from build123d import *

# Parameters (mm, degrees)
SKETCH_1_R           = 47
EXTRUDE_1_DEPTH      = 25
SKETCH_2_R           = 78
EXTRUDE_2_DEPTH      = 24
SKETCH_3_R           = 56
EXTRUDE_3_DEPTH      = 30
EXTRUDE_4_DEPTH      = 60
EXTRUDE_4_DEPTH_BACK = 60
SKETCH_4_R           = 58
SKETCH_4_R_2         = 38


with BuildPart() as part:
    # 草图1 → 凸台-拉伸1 (new body)
    with BuildSketch(Plane.XY):
        Circle(SKETCH_1_R)
    extrude(amount=-EXTRUDE_1_DEPTH)

    # 草图2 → 凸台-拉伸2 (add)
    with BuildSketch(Plane.XY):
        Circle(SKETCH_2_R)
    extrude(amount=EXTRUDE_2_DEPTH)

    # 草图3 → 凸台-拉伸3 (add)
    with BuildSketch(Plane.XY):
        Circle(SKETCH_3_R)
    extrude(amount=EXTRUDE_3_DEPTH)

    # 草图4 → 凸台-拉伸4 (add, two sides: drawn at the far end of the back side and taken through both)
    with BuildSketch(Plane(origin=(0, 0, 0), x_dir=(1, 0, 0), z_dir=(0, 1, 0)).offset(-EXTRUDE_4_DEPTH_BACK)):
        with Locations((0, -60)):
            Circle(SKETCH_4_R)
        with Locations((0, -60)):
            Circle(SKETCH_4_R_2, mode=Mode.SUBTRACT)
    extrude(amount=EXTRUDE_4_DEPTH + EXTRUDE_4_DEPTH_BACK)


solid = part.part
Build history of the part. All positions in model axes, mm. A direction names the side the tool comes from. Give positions to 0.01 mm unless a question says otherwise; leave off trailing zeros. Write each loop counter-clockwise with the first axis right and the second up, starting at its lowest first coordinate (ties: lowest second). Pieces come first, ordered by that corner, then holes. Notation, with made-up numbers: (-23, -4) - (7, -4) arc R15 ccw to (7, 22) - close; hole circle Ø11 at (84, -24.5). An arc over 180 degrees is marked (long way). Use one line per item in the form item = value. Start each with the question number.
1. Probe line 1 (X direction, y = 30.5, z = 60); line 2 (Z direction, x = 0, y = -32.5); line 3 (X direction, y = -57.5, z = 29). List the from-to ranges inside material, lowest first. Write a range as [from, to].
2. Band-saw the part on C-C on x = 0. Write the cut outline in (y, z).
3. Band-saw the part on D-D on x = -19. Write the cut outline in (y, z).
4. Drop flat-ended pins along their axis: pin 1 Ø3 at (x, y) = (-51, -4.5) entering from +Z; pin 2 Ø5 at (y, z) = (44.5, 83.5) entering from +X; pin 3 Ø3 at (y, z) = (-20, 12.5) entering from +X. Give the stop position or say it passes through.
5. 3-axis set-ups, long thin cutter, end or side, ignore diameter. For faces 1 (the face through (56, 0, 27)), 2 (the face through (-56, 0, 27)), 3 (the face through (0, 1, 30)): which of +Z, -Z, +X, -X, +Y, -Y reach the whole face in a straight line?
6. Band-saw the part on B-B on y = 0. Write the cut outline in (x, z).
7. Band-saw the part on A-A on z = 60. Write the cut outline in (x, y).
Conclusion:
q1.line_1 = [-58, -38], [38, 58]
q1.line_2 = [-25, 30], [98, 118]
q1.line_3 = [-49.02, -21.98], [21.98, 49.02]
q2.outline = (-78, 0) - (-47, 0) - (-47, -25) - (47, -25) - (47, 0) - (78, 0) - (78, 24) - (56, 24) - (56, 30) - (-56, 30) - (-56, 24) - (-78, 24) - close; (-60, 98) - (60, 98) - (60, 118) - (-60, 118) - close
q3.outline = (-75.65, 0) - (-42.99, 0) - (-42.99, -25) - (42.99, -25) - (42.99, 0) - (75.65, 0) - (75.65, 24) - (60, 24) - (60, 27.09) - (52.68, 27.09) - (52.68, 30) - (-52.68, 30) - (-52.68, 27.09) - (-60, 27.09) - (-60, 24) - (-75.65, 24) - close; (-60, 92.91) - (60, 92.91) - (60, 114.8) - (-60, 114.8) - close
q4.pin_1 = 90.23
q4.pin_2 = 54.06
q4.pin_3 = 75.77
q5.face_1 = +X
q5.face_2 = -X
q5.face_3 = +Y, -Y
q6.outline = (-78, 0) - (-47, 0) - (-47, -25) - (47, -25) - (47, 0) - (78, 0) - (78, 24) - (56, 24) - (56, 30) - (49.64, 30) arc R58 ccw (long way) to (-49.64, 30) - (-56, 30) - (-56, 24) - (-78, 24) - close; hole (-23.32, 30) - (23.32, 30) arc R38 ccw (long way) to start
q7.outline = (-58, -60) - (-38, -60) - (-38, 60) - (-58, 60) - close; (38, -60) - (58, -60) - (58, 60) - (38, 60) - close
